Job drawing, mm, ordinate dimensions from the low corner. One solid piece. A direction names the side the tool comes from. Round coordinates to 2 decimals unless told otherwise and drop trailing zeros. Loops run counter-clockwise (first coordinate to the right, second up) from the corner with the lowest first, then second, coordinate; pieces in that order, holes last.
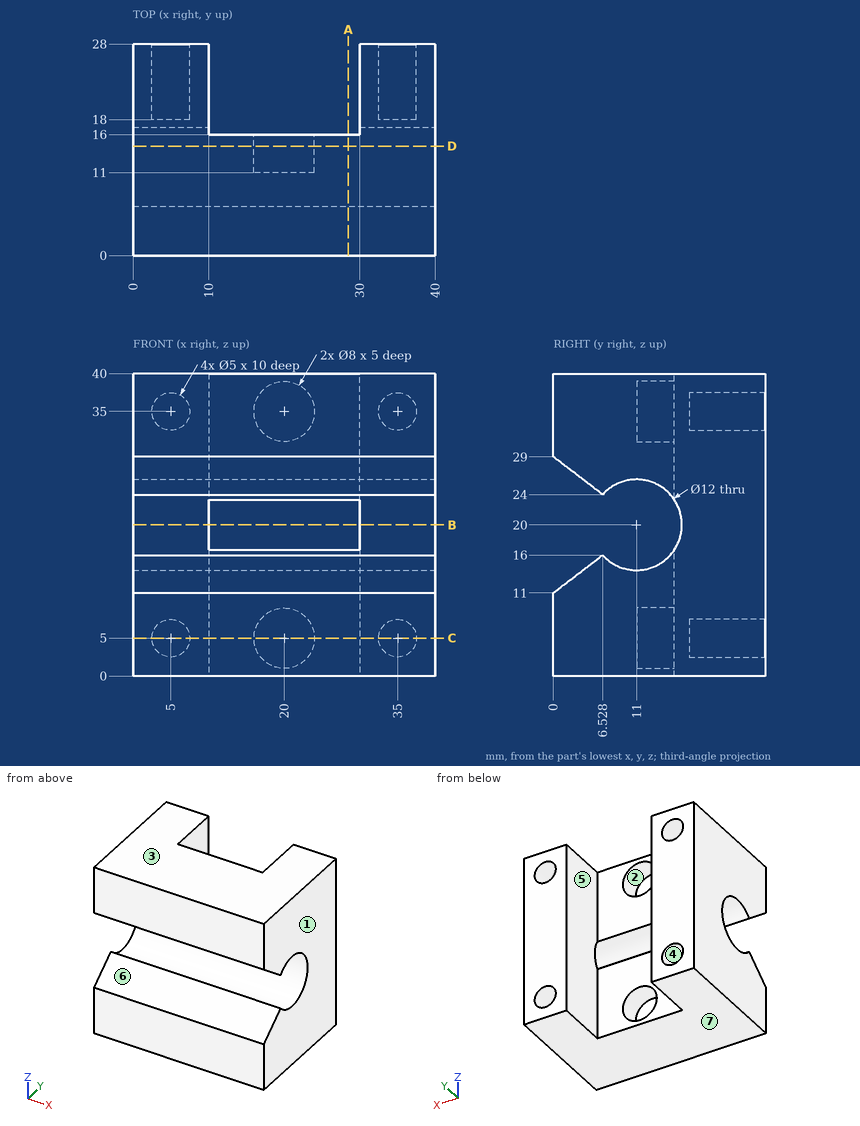
Item 1: Cut at D-D, the plane y = 14.5. Give the cut face in (x, z), plus the area to 3 significant figures.
Answers follow:
outline: (0, 0) - (40, 0) - (40, 15.13) - (0, 15.13) - close; (0, 24.87) - (40, 24.87) - (40, 40) - (0, 40) - close; hole circle Ø8 at (20, 5); hole circle Ø8 at (20, 35)
area: 1,110 mm2
Item 2: Two-plate mould, pull along X, no slides. Class the marked faces 1, 2 and 3: released by +X, released by -X, zero draft, split by the parting line, or undercut.
Answers follow:
face 1: released by +X
face 2: undercut
face 3: zero draft
Item 3: 3-axis set-ups, long thin cutter, end or side, ignore diameter. For the marked faces 4, 5, 6 and 7: which of +Z, -Z, +X, -X, +Y, -Y reach the whole face in a straight line?
Answers follow:
face 4: +Y
face 5: +Z, -Z, +Y
face 6: +X, -X, -Y
face 7: -Z, +X, -X, +Y, -Y
Item 4: Cut at C-C, the plane z = 5. Give the cut face in (x, y), plus the area to 3 significant figures.
Answers follow:
outline: (0, 0) - (40, 0) - (40, 28) - (37.5, 28) - (37.5, 18) - (32.5, 18) - (32.5, 28) - (30, 28) - (30, 16) - (24, 16) - (24, 11) - (16, 11) - (16, 16) - (10, 16) - (10, 28) - (7.5, 28) - (7.5, 18) - (2.5, 18) - (2.5, 28) - (0, 28) - close
area: 740 mm2
Item 5: Cut at B-B, the plane z = 20. Give the cut face in (x, y).
Answers follow:
outline: (0, 17) - (10, 17) - (10, 28) - (0, 28) - close; (30, 17) - (40, 17) - (40, 28) - (30, 28) - close
Item 6: Flat gauge pins, fed straight in: P1, Ø4, axis at x = 35, z = 35, coming from the +Y side; P2, Ø5, axis at x = 19, z = 9.5, coming from the +Y side; P3, Ø6.5, axis at x = 20, z = 35, coming from the +Y side. Where does each tip first touch, or does it go through?
Answers follow:
P1: stops at y = 18
P2: stops at y = 16
P3: stops at y = 11
Item 7: Cut at A-A, the plane x = 28.5. Give the cut face in (y, z).
Answers follow:
outline: (0, 0) - (16, 0) - (16, 16.68) arc R6 cw to (6.53, 16) - (0, 11) - close; (0, 29) - (6.53, 24) arc R6 cw to (16, 23.32) - (16, 40) - (0, 40) - close
Item 8: Probe line 1 (X direction, y = 23.5, z = 5); line 2 (X direction, y = 18.25, z = 22.5); line 3 (X direction, y = 12.3, z = 35). List the from-to ranges inside material, lowest first.
Answers follow:
line 1: x = 0 to 2.5, 7.5 to 10, 30 to 32.5, 37.5 to 40
line 2: x = 0 to 10, 30 to 40
line 3: x = 0 to 16, 24 to 40
